The model under review builds one solid part; all positions refer to its coordinate system, in mm. A direction names the side the tool comes from. Give positions to 0.01 mm unless a question says otherwise; leave off trailing zeros. Loops run counter-clockwise (first coordinate to the right, second up) from the corner with the lowest first, then second, coordinate; pieces in that order, holes last. Notation, with made-up numbers: M 60,44.5 L 85,44.5 A32 ccw 85,75.5 Z; hole C 39.5,3.25 d8. An arc over 180 degrees is marked long. Return JSON: item names as keys, results as strings. Group by question number.
```python
from build123d import *

# Parameters (mm, degrees)
Y_KSEKLIK_EKSTR_ZYON1_DEPTH = 35
KES_EKSTR_ZYON2_DEPTH       = 32.5
IZIM6_W                     = 20
IZIM6_H                     = 25
KES_EKSTR_ZYON3_DEPTH       = 12.5
IZIM7_R                     = 3.5
KES_EKSTR_ZYON4_DEPTH       = 12.5
IZIM8_W                     = 8
IZIM8_H                     = 15
KES_EKSTR_ZYON5_DEPTH       = 12.5


with BuildPart() as part:
    # Çizim1 → Yükseklik-Ekstrüzyon1 (new body)
    with BuildSketch(Plane(origin=(0, 0, 0), x_dir=(1, 0, 0), z_dir=(0, 1, 0))):
        Polygon((80, 0), (110.4139872, 17.348793327), (110.4139872, 60), (110.4139872, 80.241023143), (80, 80.241023143), (80, 60), (0, 60), (0, 0), align=None)
    extrude(amount=Y_KSEKLIK_EKSTR_ZYON1_DEPTH)

    # Çizim5 → Kes-Ekstrüzyon2 (cut)
    with BuildSketch(Plane(origin=(0, 0, 0), x_dir=(-1, 0, 0), z_dir=(0, -1, 0))):
        Polygon((-2.5, 2.5), (-80, 2.5), (-107.9139872, 18.34615917), (-107.9139872, 77.741023143), (-82.5, 77.741023143), (-82.5, 57.5), (-80.013539943, 57.5), (-2.5, 57.5), align=None)
    extrude(amount=-KES_EKSTR_ZYON2_DEPTH, mode=Mode.SUBTRACT)

    # Çizim6 → Kes-Ekstrüzyon3 (cut)
    with BuildSketch(Plane(origin=(19.639985559, 0, 34.430652215), x_dir=(0.8686196984341679, 0, -0.4954793835187649), z_dir=(0.4954793835187649, 0, 0.8686196984341679))):
        with Locations((86.989575875, 17.5)):
            Rectangle(IZIM6_W, IZIM6_H)
    extrude(amount=-KES_EKSTR_ZYON3_DEPTH, mode=Mode.SUBTRACT)

    # Çizim7 → Kes-Ekstrüzyon4 (cut)
    with BuildSketch(Plane(origin=(0, 0, -80.241023143), x_dir=(-1, 0, 0), z_dir=(0, 0, -1))):
        with Locations((-97.4139872, 17.5)):
            Circle(IZIM7_R)
    extrude(amount=-KES_EKSTR_ZYON4_DEPTH, mode=Mode.SUBTRACT)

    # Çizim8 → Kes-Ekstrüzyon5 (cut)
    with BuildSketch(Plane.XY):
        with Locations((66.154872496, 15.5)):
            Rectangle(IZIM8_W, IZIM8_H)
    extrude(amount=-KES_EKSTR_ZYON5_DEPTH, mode=Mode.SUBTRACT)


solid = part.part
```
(1) For probe 1 along X at (y, z) = (8.5, -56); probe 2 along Z at (x, y) = (70, 5.5); probe 3 along Y at (x, z) = (64, -11), list the stretches that pass through material, from the lowest coordinate up.
(2) Mouldability with a two-part tool opening along Y and no side actions: class faces 1 (the flat face through (95, 30, -10)), 2 (the flat face through (82.5, 16, -68)) as released by +Y, released by -Y, zero draft, split by the parting line, or undercut.
(3) Add section A-A (y = 17.5). Write out the cut boundary in (x, z), and give its area (3 significant figures).
(4) For faces 3 (the flat face through (41, 17, -60)), 4 (the flat face through (93, 16, -77.741)), 5 (the flat face through (66, 23, -1)), list the 3-axis set-ups (+Z, -Z, +X, -X, +Y, -Y) from which the entire face can be reached by the end or side of a thin tool; tool diameter is ignored.
(5) Add section B-B (x = 19.5). Write out the cut boundary in (y, z).
(6) For pin 1 (1.5 mm diameter, centred on x = 56.5, z = -29.5, fed in from -Y); pin 2 (1.2 mm diameter, centred on y = 15.5, z = -1.5, fed in from +X); pin 3 (6 mm diameter, centred on y = 15, z = -67, fed in from -X), all flat-tipped, find the tip position at first contact; note any pin that passes through.
(7) Add section D-D (z = -8). Write out the cut boundary in (x, y).
(8) Add section C-C (z = -44). Write out the cut boundary in (x, y), and give its area (3 significant figures).
Verdict:
{
 "1": {"probe 1": "x = 0 to 2.5, 107.91 to 110.41", "probe 2": "z = -60 to -57.5, -2.5 to 0", "probe 3": "y = 32.5 to 35"},
 "2": {"face 1": "undercut", "face 2": "zero draft"},
 "3": {"outline": "M 0,-60 L 80,-60 L 80,-80.24 L 93.91,-80.24 L 93.91,-77.74 L 82.5,-77.74 L 82.5,-57.5 L 2.5,-57.5 L 2.5,-2.5 L 62.15,-2.5 L 62.15,0 L 0,0 Z; M 70.15,-2.5 L 80,-2.5 L 85.45,-5.59 L 86.51,-3.72 L 80,0 L 70.15,0 Z; M 100.91,-80.24 L 110.41,-80.24 L 110.41,-17.35 L 103.89,-13.63 L 102.84,-15.46 L 107.91,-18.35 L 107.91,-77.74 L 100.91,-77.74 Z", "area": "805 mm²"},
 "4": {"face 3": "-Z, -X, +Y, -Y", "face 4": "-Y", "face 5": "+Z"},
 "5": {"outline": "M 0,-60 L 35,-60 L 35,0 L 0,0 L 0,-2.5 L 32.5,-2.5 L 32.5,-57.5 L 0,-57.5 Z"},
 "6": {"pin 1": "stops at y = 32.5", "pin 2": "stops at x = 83.68", "pin 3": "stops at x = 80"},
 "7": {"outline": "M 0,0 L 2.5,0 L 2.5,32.5 L 89.69,32.5 L 89.69,30 L 94.02,30 L 94.02,35 L 0,35 Z; M 89.69,0 L 94.02,0 L 94.02,5 L 89.69,5 Z"},
 "8": {"outline": "M 0,0 L 2.5,0 L 2.5,32.5 L 107.91,32.5 L 107.91,0 L 110.41,0 L 110.41,35 L 0,35 Z", "area": "439 mm²"}
}
